```python
from build123d import *

# Parameters (mm, degrees)
BASE_EXTRUDE_DEPTH = 54.737
SKETCH2_R          = 4.1656
HOLE_DEPTH         = 77.807285911
HOLE_PATTERN_COUNT = 3
HOLE_PATTERN_PITCH = 38.1
SLOT_DEPTH         = 77.807285911
SLOT_PATTERN_COUNT = 3
SLOT_PATTERN_PITCH = 38.1


with BuildPart() as part:
    # Sketch1 → Base Extrude (new, symmetric)
    with BuildSketch(Plane(origin=(0, 0, 0), x_dir=(0, 0, -1), z_dir=(1, 0, 0))):
        with BuildLine():
            Line((-6.35, 12.7), (-6.35, 31.75))
            ThreePointArc((-6.35, 31.75), (-4.490128061, 36.240128061), (0, 38.1))
            Line((0, 38.1), (0, 0))
            Line((0, 0), (-38.1, 0))
            ThreePointArc((-38.1, 0), (-36.240128061, 4.490128061), (-31.75, 6.35))
            Line((-31.75, 6.35), (-12.7, 6.35))
            ThreePointArc((-12.7, 6.35), (-8.209871939, 8.209871939), (-6.35, 12.7))
        make_face()
    extrude(amount=BASE_EXTRUDE_DEPTH, both=True)

    # Sketch2 → Hole (cut, through all)
    with BuildSketch(Plane.XZ):
        with Locations(Location((-38.1, 19.05, 0), (0, 0, 270))):
            Circle(SKETCH2_R)
    hole = extrude(amount=-HOLE_DEPTH, mode=Mode.SUBTRACT)

    # Hole Pattern: Hole ×3
    with Locations(*[(i * HOLE_PATTERN_PITCH, 0, 0) for i in range(1, HOLE_PATTERN_COUNT)]):
        add(hole, mode=Mode.SUBTRACT)

    # Sketch3 → Slot (cut, through all)
    with BuildSketch(Plane(origin=(0, 0, 0), x_dir=(-1, 0, 0), z_dir=(0, 0, -1))):
        with BuildLine():
            Line((42.2656, 25.4), (42.2656, 12.7))
            ThreePointArc((42.2656, 12.7), (38.1, 8.5344), (33.9344, 12.7))
            Line((33.9344, 12.7), (33.9344, 25.4))
            ThreePointArc((33.9344, 25.4), (38.1, 29.5656), (42.2656, 25.4))
        make_face()
    slot = extrude(amount=-SLOT_DEPTH, mode=Mode.SUBTRACT)

    # Slot Pattern: Slot ×3
    with Locations(*[(i * SLOT_PATTERN_PITCH, 0, 0) for i in range(1, SLOT_PATTERN_COUNT)]):
        add(slot, mode=Mode.SUBTRACT)


solid = part.part
```
Build history of the part. All positions in model axes, mm. A direction names the side the tool comes from. Round coordinates to 2 decimals unless told otherwise and drop trailing zeros. Write each loop counter-clockwise with the first axis right and the second up, starting at its lowest first coordinate (ties: lowest second). Pieces come first, ordered by that corner, then holes. Notation, with made-up numbers: (-26, 82.5) - (-4, 82.5) arc R26 cw to (-4, 117.5) - close; hole circle Ø9 at (74.25, 31.5). An arc over 180 degrees is marked (long way). Write each question's results on one line, items separated by ' | '. Start each with the question number.
Item 1: Mould opens along X. For faces 1 (the face through (0.77, 36.19, 4.54)), 2 (the face through (54.737, 13, 6)), 3 (the face through (4.166, 19, 3)) say: pulls with the +X half, pulls with the -X half, needs draft (parallel to the pull), parting line crosses it, or undercut.
Item 2: Wall check: L1, parallel to X at y = 3, z = 19; L2, parallel to Y at x = -46.5, z = 20. Give the ranges that are in metal, low to high. Write a range as [from, to].
Item 3: Which spindle directions (+Z, -Z, +X, -X, +Y, -Y) get a long thin tool onto all of the face, cutting with end or side? Do faces 4 (the face through (40.915, 3.131, 22.12)), 5 (the face through (1, 6.35, 24)), 6 (the face through (-38.008, 29.565, 3.131)). Say none if no direction does.
Item 4: Saw through at D-D (z = 4). Write the cut outline in (x, y).
Item 5: Saw through at C-C (x = -10). Write the cut outline in (y, z).
Item 6: Drop flat-ended pins along their axis: P1, Ø4, axis at x = -34, y = 16.5, coming from the +Z side; P2, Ø8, axis at x = 20.5, z = 34, coming from the +Y side; P3, Ø7.5, axis at x = 38.1, z = 19.05, coming from the -Y side; P4, Ø15, axis at x = 11.5, z = 19.5, coming from the +Y side. Give the stop position or say it passes through.
Item 7: Saw through at A-A (z = 19.05). Write the cut outline in (x, y).
Results are:
1) face 1: needs draft | face 2: pulls with the +X half | face 3: undercut
2) L1: x = [-54.74, -42.27], [-33.93, -4.17], [4.17, 33.93], [42.27, 54.74] | L2: y = [0, 6.35]
3) face 4: +Y, -Y | face 5: +Z, +X, -X, +Y | face 6: +Z, -Z
4) outline: (-54.74, 0) - (54.74, 0) - (54.74, 36.68) - (-54.74, 36.68) - close; hole (-42.27, 12.7) arc R4.17 ccw to (-33.93, 12.7) - (-33.93, 25.4) arc R4.17 ccw to (-42.27, 25.4) - close; hole (-4.17, 12.7) arc R4.17 ccw to (4.17, 12.7) - (4.17, 25.4) arc R4.17 ccw to (-4.17, 25.4) - close; hole (33.93, 12.7) arc R4.17 ccw to (42.27, 12.7) - (42.27, 25.4) arc R4.17 ccw to (33.93, 25.4) - close
5) outline: (0, 0) - (38.1, 0) arc R6.35 ccw to (31.75, 6.35) - (12.7, 6.35) arc R6.35 cw to (6.35, 12.7) - (6.35, 31.75) arc R6.35 ccw to (0, 38.1) - close
6) P1: stops at z = 6.35 | P2: stops at y = 6.35 | P3: passes through | P4: stops at y = 6.39
7) outline: (-54.74, 0) - (-42.27, 0) - (-42.27, 6.35) - (-54.74, 6.35) - close; (-33.93, 0) - (-4.17, 0) - (-4.17, 6.35) - (-33.93, 6.35) - close; (4.17, 0) - (33.93, 0) - (33.93, 6.35) - (4.17, 6.35) - close; (42.27, 0) - (54.74, 0) - (54.74, 6.35) - (42.27, 6.35) - close
